from build123d import *

# Parameters (mm, degrees)
SKETCH023_W     = 98
SKETCH023_H     = 107
PAD018_DEPTH    = 44
SKETCH024_W     = 92.4
SKETCH024_H     = 101.4
POCKET003_DEPTH = 42
SKETCH025_W     = 2.8
SKETCH025_H     = 52
POCKET004_DEPTH = 6.2
SKETCH026_W     = 87
SKETCH026_H     = 54
POCKET005_DEPTH = 2
SKETCH027_W     = 7
SKETCH027_H     = 12
PAD019_DEPTH    = 2
SKETCH028_W     = 7
SKETCH028_H     = 12
PAD020_DEPTH    = 2
SKETCH029_R     = 1.6
POCKET006_DEPTH = 98.001
SKETCH030_R     = 3.2
POCKET007_DEPTH = 2.2
SKETCH031_R     = 3.2
POCKET008_DEPTH = 2.2
SKETCH032_W     = 9.4
SKETCH032_H     = 3.8
SKETCH032_W_2   = 7.8
SKETCH032_H_2   = 3
SKETCH032_W_3   = 7
SKETCH032_H_3   = 7
POCKET009_DEPTH = 2.8
SKETCH033_W     = 13.4
SKETCH033_H     = 6
POCKET010_DEPTH = 2.8
SKETCH040_R     = 1.2
POCKET011_DEPTH = 2
SKETCH043_W     = 8
SKETCH043_H     = 6
POCKET013_DEPTH = 5
SKETCH044_W     = 20
SKETCH044_H     = 6
POCKET014_DEPTH = 0.6
SKETCH045_W     = 21
SKETCH045_H     = 7
POCKET015_DEPTH = 0.6
CHAMFER_SIZE    = 1
SKETCH047_W     = 15.4
SKETCH047_H     = 17
POCKET016_DEPTH = 0.6
CHAMFER001_SIZE = 1.9
SKETCH057_R     = 1.2
POCKET021_DEPTH = 3
POCKET023_DEPTH = 0.6
FILLET_R        = 0.4


with BuildPart() as part:
    # Sketch023 → Pad018 (new body)
    with BuildSketch(Plane.XY.offset(27)):
        with Locations((0.5, 0.5)):
            Rectangle(SKETCH023_W, SKETCH023_H)
    extrude(amount=-PAD018_DEPTH)

    # Sketch024 (on Face6 of Pad018) → Pocket003 (cut)
    with BuildSketch(Plane(origin=(0, 0, -17), x_dir=(1, 0, 0), z_dir=(0, 0, -1))):
        with Locations((0.5, -0.5)):
            Rectangle(SKETCH024_W, SKETCH024_H)
    extrude(amount=-POCKET003_DEPTH, mode=Mode.SUBTRACT)

    # Sketch025 (on Face5 of Pocket003) → Pocket004 (cut)
    with BuildSketch(Plane(origin=(0, 0, -17), x_dir=(1, 0, 0), z_dir=(0, 0, -1))):
        with Locations((-47.1, 0)):
            Rectangle(SKETCH025_W, SKETCH025_H)
        with Locations((48.1, 0)):
            Rectangle(SKETCH025_W, SKETCH025_H)
    extrude(amount=-POCKET004_DEPTH, mode=Mode.SUBTRACT)

    # Sketch026 (on Face4 of Pocket004) → Pocket005 (cut)
    with BuildSketch(Plane.XY.offset(27)):
        with Locations((1, 22)):
            Rectangle(SKETCH026_W, SKETCH026_H)
    extrude(amount=-POCKET005_DEPTH, mode=Mode.SUBTRACT)

    # Sketch027 (on Face18 of Pocket005) → Pad019 (join)
    with BuildSketch(Plane.YZ.offset(-45.7)):
        with Locations((-46.7, -11)):
            Rectangle(SKETCH027_W, SKETCH027_H)
        with Locations((47.7, -11)):
            Rectangle(SKETCH027_W, SKETCH027_H)
    extrude(amount=PAD019_DEPTH)

    # Sketch028 (on Face21 of Pad019) → Pad020 (join)
    with BuildSketch(Plane(origin=(46.7, 0, 0), x_dir=(0, -1, 0), z_dir=(-1, 0, 0))):
        with Locations((-47.7, -11)):
            Rectangle(SKETCH028_W, SKETCH028_H)
        with Locations((46.7, -11)):
            Rectangle(SKETCH028_W, SKETCH028_H)
    extrude(amount=PAD020_DEPTH)

    # Sketch029 (on Face3 of Pad020) → Pocket006 (cut, through all)
    with BuildSketch(Plane.YZ.offset(49.5)):
        with Locations((-47, -12)):
            Circle(SKETCH029_R)
        with Locations((48, -12)):
            Circle(SKETCH029_R)
    extrude(amount=-POCKET006_DEPTH, mode=Mode.SUBTRACT)

    # Sketch030 (on Face3 of Pocket006) → Pocket007 (cut)
    with BuildSketch(Plane.YZ.offset(49.5)):
        with Locations((48, -12)):
            Circle(SKETCH030_R)
        with Locations((-47, -12)):
            Circle(SKETCH030_R)
    extrude(amount=-POCKET007_DEPTH, mode=Mode.SUBTRACT)

    # Sketch031 (on Face2 of Pocket007) → Pocket008 (cut)
    with BuildSketch(Plane(origin=(-48.5, 0, 0), x_dir=(0, -1, 0), z_dir=(-1, 0, 0))):
        with Locations((47, -12)):
            Circle(SKETCH031_R)
        with Locations((-48, -12)):
            Circle(SKETCH031_R)
    extrude(amount=-POCKET008_DEPTH, mode=Mode.SUBTRACT)

    # Sketch032 (on Face2 of Pocket008) → Pocket009 (cut)
    with BuildSketch(Plane(origin=(-48.5, 0, 0), x_dir=(0, -1, 0), z_dir=(-1, 0, 0))):
        with Locations((-39.5, 16.3)):
            Rectangle(SKETCH032_W, SKETCH032_H)
        with Locations((-37.5, 3.3)):
            Rectangle(SKETCH032_W, SKETCH032_H)
        with Locations((-25.3, 2.9)):
            Rectangle(SKETCH032_W_2, SKETCH032_H_2)
        with Locations((30.1, 14.1)):
            Rectangle(SKETCH032_W_3, SKETCH032_H_3)
    extrude(amount=-POCKET009_DEPTH, mode=Mode.SUBTRACT)

    # Sketch033 (on Face6 of Pocket009) → Pocket010 (cut)
    with BuildSketch(Plane.XZ.offset(53)):
        with Locations((-0.4, -4)):
            Rectangle(SKETCH033_W, SKETCH033_H)
    extrude(amount=-POCKET010_DEPTH, mode=Mode.SUBTRACT)

    # Sketch040 (on Face4 of Pocket010) → Pocket011 (cut)
    with BuildSketch(Plane.XY.offset(27)):
        with Locations((28, -10)):
            Circle(SKETCH040_R)
        with Locations((34, -10)):
            Circle(SKETCH040_R)
        with Locations((40, -10)):
            Circle(SKETCH040_R)
        with BuildLine():
            Line((-18, -22.6), (-7.4, -22.6))
            Line((-7.4, -22.6), (-7.4, -15.5))
            ThreePointArc((-3, -11.1), (-6.11127, -12.38873), (-7.4, -15.5))
            Line((-3, -11.1), (3, -11.1))
            ThreePointArc((7.4, -15.5), (6.11127, -12.38873), (3, -11.1))
            Line((7.4, -15.5), (7.4, -22.6))
            Line((7.4, -22.6), (18, -22.6))
            ThreePointArc((22.4, -27), (21.11127, -23.88873), (18, -22.6))
            Line((22.4, -27), (22.4, -30.5))
            ThreePointArc((18, -34.9), (21.11127, -33.61127), (22.4, -30.5))
            Line((18, -34.9), (7.4, -34.9))
            Line((7.4, -34.9), (7.4, -42))
            ThreePointArc((3, -46.4), (6.11127, -45.11127), (7.4, -42))
            Line((3, -46.4), (-3, -46.4))
            ThreePointArc((-7.4, -42), (-6.11127, -45.11127), (-3, -46.4))
            Line((-7.4, -42), (-7.4, -34.9))
            Line((-7.4, -34.9), (-18, -34.9))
            ThreePointArc((-22.4, -30.5), (-21.11127, -33.61127), (-18, -34.9))
            Line((-22.4, -30.5), (-22.4, -27))
            ThreePointArc((-18, -22.6), (-21.11127, -23.88873), (-22.4, -27))
        make_face()
    extrude(amount=-POCKET011_DEPTH, mode=Mode.SUBTRACT)

    # Sketch043 (on Face3 of Pocket011) → Pocket013 (cut)
    with BuildSketch(Plane.YZ.offset(49.5)):
        with Locations((-38.6, -2)):
            Rectangle(SKETCH043_W, SKETCH043_H)
    extrude(amount=-POCKET013_DEPTH, mode=Mode.SUBTRACT)

    # Sketch044 (on Face69 of Pocket013) → Pocket014 (cut)
    with BuildSketch(Plane(origin=(46.7, 0, 0), x_dir=(0, -1, 0), z_dir=(-1, 0, 0))):
        with Locations((38.6, -2)):
            Rectangle(SKETCH044_W, SKETCH044_H)
    extrude(amount=-POCKET014_DEPTH, mode=Mode.SUBTRACT)

    # Sketch045 (on Face66 of Pocket014) → Pocket015 (cut)
    with BuildSketch(Plane.YZ.offset(-45.7)):
        with Locations((-30.1, 14.1)):
            Rectangle(SKETCH045_W, SKETCH045_H)
    extrude(amount=-POCKET015_DEPTH, mode=Mode.SUBTRACT)

    # Chamfer
    chamfer_edges = [part.edges().sort_by_distance(p)[0] for p in [
        (-42.5, 22, 27),
        (1, 49, 27),
        (44.5, 22, 27),
        (1, -5, 27),
    ]]
    chamfer(chamfer_edges, length=CHAMFER_SIZE)

    # Sketch047 (on Face81 of Chamfer) → Pocket016 (cut)
    with BuildSketch(Plane(origin=(0, -50.2, 0), x_dir=(-1, 0, 0), z_dir=(0, 1, 0))):
        with Locations((0.4, -8.5)):
            Rectangle(SKETCH047_W, SKETCH047_H)
    extrude(amount=-POCKET016_DEPTH, mode=Mode.SUBTRACT)

    # Chamfer001
    chamfer001_edges = [part.edges().sort_by_distance(p)[0] for p in [
        (-43.7, -46.7, -5),
        (-43.7, 47.7, -5),
        (44.7, 47.7, -5),
        (44.7, -46.7, -5),
    ]]
    chamfer(chamfer001_edges, length=CHAMFER001_SIZE)

    # Sketch057 (on Face90 of Chamfer001) → Pocket021 (cut)
    with BuildSketch(Plane.XZ.offset(53)):
        with Locations((25, -14)):
            Circle(SKETCH057_R)
        with Locations((30, -14)):
            Circle(SKETCH057_R)
    extrude(amount=-POCKET021_DEPTH, mode=Mode.SUBTRACT)

    # Sketch059 (on Face15 of Pocket021) → Pocket023 (cut)
    with BuildSketch(Plane(origin=(-48.5, 0, 0), x_dir=(0, -1, 0), z_dir=(-1, 0, 0))):
        with BuildLine():
            Line((-44.2, 21.6), (-34.8, 21.6))
            ThreePointArc((-31.4, 18.2), (-32.395837, 20.604163), (-34.8, 21.6))
            Line((-31.4, 11.2), (-31.4, 18.2))
            ThreePointArc((-31.4, 11.2), (-30.404163, 8.795837), (-28, 7.8))
            Line((-21.4, 7.8), (-28, 7.8))
            ThreePointArc((-18, 4.4), (-18.995837, 6.804163), (-21.4, 7.8))
            Line((-18, 4.4), (-18, 1.4))
            ThreePointArc((-21.4, -2), (-18.995837, -1.004163), (-18, 1.4))
            Line((-21.4, -2), (-44.2, -2))
            ThreePointArc((-47.6, 1.4), (-46.604163, -1.004163), (-44.2, -2))
            Line((-47.6, 1.4), (-47.6, 18.2))
            ThreePointArc((-44.2, 21.6), (-46.604163, 20.604163), (-47.6, 18.2))
        make_face()
    extrude(amount=-POCKET023_DEPTH, mode=Mode.SUBTRACT)

    # Fillet
    fillet_edges = [part.edges().sort_by_distance(p)[0] for p in [
        (-48.5, 32.8, -2),
        (-48.5, 18.995837, -1.004163),
        (-48.5, 18, 2.9),
        (-48.5, 18.995837, 6.804163),
        (-48.5, 24.7, 7.8),
        (-48.5, 30.404163, 8.795837),
        (-48.5, 31.4, 14.7),
        (-48.5, 32.395837, 20.604163),
        (-48.5, 39.5, 21.6),
        (-48.5, 46.604163, 20.604163),
        (-48.5, 47.6, 9.8),
        (-48.5, 46.604163, -1.004163),
    ]]
    fillet(fillet_edges, radius=FILLET_R)


solid = part.part
Read the model definition and answer for the solid it produces. Units are mm, in the model's axes. A direction names the side the tool comes from. Round coordinates to 2 decimals unless told otherwise and drop trailing zeros. Order: outer loops, then holes, each group sorted by start corner. A loop starts at its lowest first (then second) coordinate and runs counter-clockwise, first axis right, second up. Notation, with made-up numbers: (41, 75.5) - (81, 75.5) arc R7 ccw to (81, 85.5) - close; hole circle Ø4 at (-22.75, 40.25). An arc over 180 degrees is marked (long way). Use one line per item in the form item = value. Start each with the question number.
(1) For faces 1 (the face through (-47, -30, 10.6)), 2 (the face through (6.077, -45.145, 26.014)), 3 (the face through (44.7, 46, -12)), 4 (the face through (-47.415, 46.523, -14.839)), determine the directions among +Z, -Z, +X, -X, +Y, -Y from which every point of the face is accessible in a straight line to the end or side of a thin tool.
(2) Find the intervals of material crossed by line 1 along Y through (x, z) = (11.5, 25.5); line 2 along X through (y, z) = (20, 3.5); line 3 along X through (y, z) = (-26, 4), in increasing order. Write a range as from..to.
(3) The part is cut by section D-D (x = -35). Give the vertices of the cut face in (y, z), then the cut area to 3 significant figures.
(4) The part is cut by section C-C (y = 11.5). Give the vertices of the cut face in (x, z), then the cut area to 3 significant figures.
(5) The part is cut by section B-B (x = -11). Give the vertices of the cut face in (y, z).
(6) The part is cut by section A-A (y = 36.5). Give the vertices of the cut face in (x, z), then the cut area to 3 significant figures.
(7) Flat-ended cylindrical pins translate along their axes: pin 1 Ø1.9 at (y, z) = (-47, -10.5) entering from -X; pin 2 Ø10 at (y, z) = (48, -12) entering from -X. Find the tip coordinate at first contact, or state that the pin passes through.
(8) Determine the mould class of faces 5 (the face through (-47.9, 36, 7)), 6 (the face through (-47.415, -48.477, -14.839)), 7 (the face through (48, -38, 1)) for opening direction X: +X half, -X half, draft (parallel to the pull), parting line (faces both ways), or undercut.
Checked values:
q1.face_1 = none
q1.face_2 = +Z, -Z
q1.face_3 = -Z
q1.face_4 = -X
q2.line_1 = -53..-34.9, -22.6..-5, 49..54
q2.line_2 = -47.9..-45.7, 46.7..49.5
q2.line_3 = -48.5..-45.7, 46.7..49.5
q3.outline = (-53, -17) - (-50.2, -17) - (-50.2, 25) - (-5, 25) - (-5, 26) - (-6, 27) - (-53, 27) - close; (49, 25) - (51.2, 25) - (51.2, -17) - (54, -17) - (54, 27) - (50, 27) - (49, 26) - close
q3.area = 340 mm^2
q4.outline = (-48.5, -10.8) - (-45.7, -10.8) - (-45.7, 25) - (-42.5, 25) - (-42.5, 26) - (-43.5, 27) - (-48.5, 27) - close; (44.5, 25) - (46.7, 25) - (46.7, -10.8) - (49.5, -10.8) - (49.5, 27) - (45.5, 27) - (44.5, 26) - close
q4.area = 221 mm^2
q5.outline = (-53, -17) - (-50.2, -17) - (-50.2, 25) - (-34.9, 25) - (-34.9, 27) - (-53, 27) - close; (-22.6, 25) - (-5, 25) - (-5, 26) - (-6, 27) - (-22.6, 27) - close; (49, 25) - (51.2, 25) - (51.2, -17) - (54, -17) - (54, 27) - (50, 27) - (49, 26) - close
q6.outline = (-48.5, -17) - (-45.7, -17) - (-45.7, 1.4) - (-47.9, 1.4) - (-47.9, -2) - (-48.1, -2) arc R0.4 ccw to (-48.5, -2.4) - close; (-48.5, 22) arc R0.4 ccw to (-48.1, 21.6) - (-47.9, 21.6) - (-47.9, 18.2) - (-45.7, 18.2) - (-45.7, 25) - (-42.5, 25) - (-42.5, 26) - (-43.5, 27) - (-48.5, 27) - close; (-47.9, 5.2) - (-45.7, 5.2) - (-45.7, 14.4) - (-47.9, 14.4) - close; (44.5, 25) - (46.7, 25) - (46.7, -17) - (49.5, -17) - (49.5, 27) - (45.5, 27) - (44.5, 26) - close
q6.area = 225 mm^2
q7.pin_1 = -46.3
q7.pin_2 = -48.5
q8.face_5 = -X half
q8.face_6 = draft
q8.face_7 = undercut
